Check sheet for the modelled part. Datum: model origin and axes. Units: mm. Face numbers are marked on the shaded views. A direction names the side the tool comes from. Round coordinates to 2 decimals unless told otherwise and drop trailing zeros. Write each loop counter-clockwise with the first axis right and the second up, starting at its lowest first coordinate (ties: lowest second). Pieces come first, ordered by that corner, then holes. Notation, with made-up numbers: M 79.25,33.5 L 90.25,33.5 A13 ccw 90.25,46.5 Z; hole C -17,33 d7. An arc over 180 degrees is marked long. Answer in a Markdown table with one row per item.
```python
from build123d import *

# Parameters (mm, degrees)
BOSS_EXTRUDE1_DEPTH     = 530
SKETCH2_R               = 22.5
CUT_EXTRUDE1_DEPTH      = 1
CUT_EXTRUDE1_DEPTH_BACK = 530.3
SKETCH3_W               = 70
SKETCH3_H               = 59
CUT_EXTRUDE2_DEPTH      = 220


with BuildPart() as part:
    # Sketch1 → Boss-Extrude1 (new body)
    with BuildSketch(Plane.XY):
        Polygon((-248.875659786, -247.380437864), (-278.875659786, -247.380437864), (-278.875659786, 281.919562136), (250.424340214, 281.919562136), (250.424340214, -247.380437864), (220.424340214, -247.380437864), (220.424340214, 251.919562136), (-248.875659786, 251.919562136), align=None)
    extrude(amount=BOSS_EXTRUDE1_DEPTH)

    # Sketch2 → Cut-Extrude1 (cut, two sides)
    with BuildSketch(Plane(origin=(250.424340214, 0, 0), x_dir=(0, 0, -1), z_dir=(1, 0, 0))) as cut_extrude1_sk:
        with Locations((-170, -82.380437864)):
            Circle(SKETCH2_R)
    extrude(amount=CUT_EXTRUDE1_DEPTH, mode=Mode.SUBTRACT)
    extrude(cut_extrude1_sk.sketch, amount=-CUT_EXTRUDE1_DEPTH_BACK, mode=Mode.SUBTRACT)

    # Sketch3 → Cut-Extrude2 (cut)
    with BuildSketch(Plane.ZY.offset(278.875659786)):
        with Locations((335, -216.880437864)):
            Rectangle(SKETCH3_W, SKETCH3_H)
    extrude(amount=-CUT_EXTRUDE2_DEPTH, mode=Mode.SUBTRACT)


solid = part.part
```
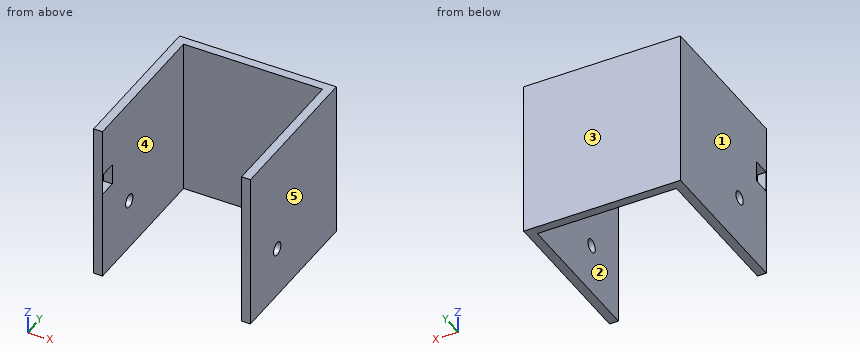
1. Scan lines: L1, parallel to Y at x = 243, z = 170; L2, parallel to X at y = -68.5, z = 401.5; L3, parallel to Y at x = -115.5, z = 441. Record each from-to range of solid material in increasing order.
Found:
| item | result |
|---|---|
| L1 | y = -247.38 to -104.88, -59.88 to 281.92 |
| L2 | x = -278.88 to -248.88, 220.42 to 250.42 |
| L3 | y = 251.92 to 281.92 |
2. Draft check along X on the marked faces 3, 4 and 5. Enter one of: +X half, -X half, draft (parallel to the pull), parting line (faces both ways), or undercut.
Found:
| item | result |
|---|---|
| face 3 | draft |
| face 4 | undercut |
| face 5 | +X half |
3. Section check C-C, the plane z = 443.5. Record the cut outline in (x, y).
Found:
| item | result |
|---|---|
| outline | M -278.88,-247.38 L -248.88,-247.38 L -248.88,251.92 L 220.42,251.92 L 220.42,-247.38 L 250.42,-247.38 L 250.42,281.92 L -278.88,281.92 Z |
4. Section check A-A, the plane z = 170. Record the cut outline in (x, y), and give its area (3 significant figures).
Found:
| item | result |
|---|---|
| outline | M -278.88,-247.38 L -248.88,-247.38 L -248.88,-104.88 L -278.88,-104.88 Z; M -278.88,-59.88 L -248.88,-59.88 L -248.88,251.92 L 220.42,251.92 L 220.42,-59.88 L 250.42,-59.88 L 250.42,281.92 L -278.88,281.92 Z; M 220.42,-247.38 L 250.42,-247.38 L 250.42,-104.88 L 220.42,-104.88 Z |
| area | 43,100 mm2 |
5. Section check B-B, the plane y = 226. Record the cut outline in (x, z).
Found:
| item | result |
|---|---|
| outline | M -278.88,0 L -248.88,0 L -248.88,530 L -278.88,530 Z; M 220.42,0 L 250.42,0 L 250.42,530 L 220.42,530 Z |
6. Go/stop test with a flat-tipped pin: pin 1 (5 mm diameter, centred on x = 197, z = 360, fed in from -Y). Record where the tip stops, or that it passes through.
Found:
| item | result |
|---|---|
| pin 1 | stops at y = 251.92 |
7. Access from +Z, -Z, +X, -X, +Y, -Y to the whole of each face (thin tool, end or side, straight path). Record for the marked faces 1 and 2.
Found:
| item | result |
|---|---|
| face 1 | +Z, -Z, -X, +Y, -Y |
| face 2 | +Z, -Z, -Y |
8. Section check D-D, the plane x = 145. Record the cut outline in (y, z).
Found:
| item | result |
|---|---|
| outline | M 251.92,0 L 281.92,0 L 281.92,530 L 251.92,530 Z |
